from build123d import *

# Parameters (mm, degrees)
BOSS_EXTRUDE1_DEPTH     = 45
BOSS_EXTRUDE2_DEPTH     = 24
CUT_EXTRUDE1_DEPTH      = 89.374204381
CUT_EXTRUDE1_DEPTH_BACK = 89.374204381
SKETCH3_W               = 16
SKETCH3_H               = 25
SKETCH4_R               = 20
CUT_EXTRUDE2_DEPTH      = 100.60923652
SKETCH5_W               = 16
SKETCH5_H               = 45
CUT_EXTRUDE3_DEPTH      = 14


with BuildPart() as part:
    # Sketch1 → Boss-Extrude1 (new, symmetric)
    with BuildSketch(Plane.XY):
        Polygon((-32, 0), (-13, 0), (-13, 14), (13, 14), (13, 0), (32, 0), (32, 32), (-32, 32), align=None)
    extrude(amount=BOSS_EXTRUDE1_DEPTH, both=True)

    # Sketch2 → Boss-Extrude2 (add, symmetric)
    with BuildSketch(Plane(origin=(0, 0, 0), x_dir=(0, 0, -1), z_dir=(1, 0, 0))):
        Polygon((-45, 32), (45, 32), (30, 69), (-30, 69), align=None)
    extrude(amount=BOSS_EXTRUDE2_DEPTH, both=True)

    # Sketch3 → Cut-Extrude1 (cut, two sides: drawn at the far end of the back side and taken through both)
    with BuildSketch(Plane.XY.offset(-CUT_EXTRUDE1_DEPTH_BACK)):
        with Locations((0, 56.5)):
            Rectangle(SKETCH3_W, SKETCH3_H)
    extrude(amount=CUT_EXTRUDE1_DEPTH + CUT_EXTRUDE1_DEPTH_BACK, mode=Mode.SUBTRACT)

    # Sketch4 → Cut-Extrude2 (cut, through all)
    with BuildSketch(Plane(origin=(24, 0, 0), x_dir=(0, 0, -1), z_dir=(1, 0, 0))):
        with Locations((0, 69)):
            Circle(SKETCH4_R)
    extrude(amount=-CUT_EXTRUDE2_DEPTH, mode=Mode.SUBTRACT)

    # Sketch5 → Cut-Extrude3 (cut, symmetric)
    with BuildSketch(Plane.XY):
        with Locations((-24, 46.5)):
            Rectangle(SKETCH5_W, SKETCH5_H)
        with Locations((24, 46.5)):
            Rectangle(SKETCH5_W, SKETCH5_H)
    extrude(amount=CUT_EXTRUDE3_DEPTH, both=True, mode=Mode.SUBTRACT)


solid = part.part
Source: CAD feature listing. Evaluate the final solid. Frame: model axes, mm. A direction names the side the tool comes from. Coordinates: 2 decimals unless noted, no trailing zeros. Loops run counter-clockwise (first coordinate to the right, second up) from the corner with the lowest first, then second, coordinate; pieces in that order, holes last. Notation, with made-up numbers: (80.5, -28) - (100.5, -28) arc R11 ccw to (100.5, -8) - close; hole circle Ø4 at (69, 49). An arc over 180 degrees is marked (long way). One line per item, written item: value. Start each with the question number.
1. Set-up query: faces 4 (the flat face through (28, 32, -29)), 5 (the flat face through (-21, 36, 14)), 6 (the flat face through (22, 36, -14)). Return all of +Z, -Z, +X, -X, +Y, -Y with unobstructed straight access to the full face (end or side cutting, diameter ignored); none if empty.
2. Section D-D (z = 0). Return the cut outline in (x, y), and give its area (3 significant figures).
3. Mould query, pull axis X, two halves, no side actions, for faces 1 (the flat face through (-16, 36, 0)), 2 (the flat face through (8, 48, -1)), 3 (the flat face through (32, 16, 1)). Classes: pulls with the +X half, pulls with the -X half, needs draft (parallel to the pull), parting line crosses it, or undercut.
4. Section C-C (x = 0.5). Return the cut outline in (y, z), and give its area (3 significant figures).
5. Section B-B (y = 60.5). Return the cut outline in (x, z), and give its area (3 significant figures).
6. Section A-A (y = 5). Return the cut outline in (x, z).
7. Ray query, L1, parallel to X at y = 10.5, z = -38; L2, parallel to X at y = 54.5, z = -24.5; L3, parallel to Y at x = 26, z = -16. Return the intervals inside material, ascending.
8. Contact query for flat-ended pins moving along their axis: P1, Ø1.5, axis at x = 20.5, y = 37.5, coming from the +Z side; P2, Ø15.5, axis at y = 49.5, z = 24.5, coming from the +X side; P3, Ø25, axis at y = 45, z = -31.5, coming from the -X side; P4, Ø3, axis at x = -5, y = 11.5, coming from the +Z side. Output: stop coordinate, or through.
Verdict:
1. face 4: +Z, -Z, +X, +Y
1. face 5: -X, +Y
1. face 6: +X, +Y
2. outline: (-32, 0) - (-13, 0) - (-13, 14) - (13, 14) - (13, 0) - (32, 0) - (32, 24) - (16, 24) - (16, 49) - (8, 49) - (8, 44) - (-8, 44) - (-8, 49) - (-16, 49) - (-16, 24) - (-32, 24) - close
2. area: 1,890 mm2
3. face 1: pulls with the -X half
3. face 2: undercut
3. face 3: pulls with the +X half
4. outline: (14, -45) - (32, -45) - (44, -40.14) - (44, 40.14) - (32, 45) - (14, 45) - close
4. area: 2,640 mm2
5. outline: (-24, -33.45) - (-8, -33.45) - (-8, -18.1) - (-24, -18.1) - close; (-24, 18.1) - (-8, 18.1) - (-8, 33.45) - (-24, 33.45) - close; (8, -33.45) - (24, -33.45) - (24, -18.1) - (8, -18.1) - close; (8, 18.1) - (24, 18.1) - (24, 33.45) - (8, 33.45) - close
5. area: 982 mm2
6. outline: (-32, -45) - (-13, -45) - (-13, 45) - (-32, 45) - close; (13, -45) - (32, -45) - (32, 45) - (13, 45) - close
7. L1: x = -32 to -13, 13 to 32
7. L2: x = -24 to -8, 8 to 24
7. L3: y = 0 to 32
8. P1: stops at z = 43.07
8. P2: stops at x = 24
8. P3: stops at x = -24
8. P4: passes through
